Design review of the part built by this model. Coordinates are the model's own, in mm. A direction names the side the tool comes from. Coordinates: 2 decimals unless noted, no trailing zeros. Loops run counter-clockwise (first coordinate to the right, second up) from the corner with the lowest first, then second, coordinate; pieces in that order, holes last. Notation, with made-up numbers: (27.25, -2.5) -> (35.25, -2.5) arc R21 cw to (35.25, 4.5) -> close; hole circle Ø4 at (-2.5, 21.25). An arc over 180 degrees is marked (long way). Answer in a Markdown table with one row per item.
```python
from build123d import *

# Parameters (mm, degrees)
SKETCH1_R               = 63.5
BOSS_EXTRUDE1_DEPTH     = 25.4
SKETCH2_R               = 38.1
CUT_EXTRUDE1_DEPTH      = 12.7
BOSS_EXTRUDE2_DEPTH     = 50.8
SKETCH5_R               = 3.175
CUT_EXTRUDE2_DEPTH      = 1
CUT_EXTRUDE2_DEPTH_BACK = 77.2
SKETCH8_R               = 3.175
CUT_EXTRUDE3_DEPTH      = 15.24
SKETCH7_R               = 3.175
CUT_EXTRUDE5_DEPTH      = 15.24
SKETCH6_R               = 3.175
CUT_EXTRUDE6_DEPTH      = 15.24


with BuildPart() as part:
    # Sketch1 → Boss-Extrude1 (new body)
    with BuildSketch(Plane(origin=(0, 0, 0), x_dir=(1, 0, 0), z_dir=(0, 1, 0))):
        Circle(SKETCH1_R)
    extrude(amount=BOSS_EXTRUDE1_DEPTH)

    # Sketch2 → Cut-Extrude1 (cut)
    with BuildSketch(Plane(origin=(0, 25.4, 0), x_dir=(1, 0, 0), z_dir=(0, 1, 0))):
        Circle(SKETCH2_R)
    extrude(amount=-CUT_EXTRUDE1_DEPTH, mode=Mode.SUBTRACT)

    # Sketch4 → Boss-Extrude2 (add)
    with BuildSketch(Plane.XZ):
        Polygon((50.8, -29.329393675), (0, 58.65878735), (-50.8, -29.329393675), align=None)
    extrude(amount=BOSS_EXTRUDE2_DEPTH)

    # Sketch5 → Cut-Extrude2 (cut, two sides)
    with BuildSketch(Plane(origin=(0, 25.4, 0), x_dir=(1, 0, 0), z_dir=(0, 1, 0))) as cut_extrude2_sk:
        with Locations((0, 50.8)):
            Circle(SKETCH5_R)
        with Locations((43.994090512, -25.4)):
            Circle(SKETCH5_R)
        with Locations((-43.994090512, -25.4)):
            Circle(SKETCH5_R)
    extrude(amount=CUT_EXTRUDE2_DEPTH, mode=Mode.SUBTRACT)
    extrude(cut_extrude2_sk.sketch, amount=-CUT_EXTRUDE2_DEPTH_BACK, mode=Mode.SUBTRACT)

    # Sketch8 → Cut-Extrude3 (cut)
    with BuildSketch(Plane(origin=(-25.4, 0, 14.664696837), x_dir=(0.5, 0, 0.866025404), z_dir=(-0.866025404, 0, 0.5))):
        with Locations((0, -25.4)):
            Circle(SKETCH8_R)
    extrude(amount=-CUT_EXTRUDE3_DEPTH, mode=Mode.SUBTRACT)

    # Sketch7 → Cut-Extrude5 (cut)
    with BuildSketch(Plane(origin=(3.754579306, 0, -29.329393675), x_dir=(1, 0, 0), z_dir=(0, 0, 1))):
        with Locations((-3.754579306, -25.4)):
            Circle(SKETCH7_R)
    extrude(amount=CUT_EXTRUDE5_DEPTH, mode=Mode.SUBTRACT)

    # Sketch6 → Cut-Extrude6 (cut)
    with BuildSketch(Plane(origin=(25.4, 0, 14.664696837), x_dir=(0.5, 0, -0.866025404), z_dir=(0.866025404, 0, 0.5))):
        with Locations((0, -25.4)):
            Circle(SKETCH6_R)
    extrude(amount=-CUT_EXTRUDE6_DEPTH, mode=Mode.SUBTRACT)


solid = part.part
```
(1) Draft analysis for pull direction Z (two halves, no side actions). For faces 1 (the flat face through (27.3, 25.4, 27.3)), 2 (the flat face through (-12.22, -25.36, 7.01)), 3 (the cylindrical face through (-13.77, 12.52, 61.99)), 4 (the flat face through (-1, -31, -29.329)), state which applies: pulls with the +Z half, pulls with the -Z half, needs draft (parallel to the pull), parting line crosses it, or undercut.
Evaluation:
| item | result |
|---|---|
| face 1 | needs draft |
| face 2 | undercut |
| face 3 | parting line crosses it |
| face 4 | pulls with the -Z half |
(2) Take a section at C-C on y = -45.5. Give the boundary of the cut face in (x, z), and give its area (3 significant figures).
Evaluation:
| item | result |
|---|---|
| outline | (-50.8, -29.33) -> (50.8, -29.33) -> (0, 58.66) -> close |
| area | 4,470 mm² |
(3) For pin 1 (10 mm diameter, centred on x = 0, z = -50.8, fed in from -Y); pin 2 (8 mm diameter, centred on y = 6.5, z = 15.5, fed in from -X); pin 3 (12 mm diameter, centred on x = 30, y = 12.5, fed in from -Z); pin 4 (10 mm diameter, centred on x = -43.99, z = 25.4, fed in from +Y), all flat-tipped, find the tip position at first contact; note any pin that passes through.
Evaluation:
| item | result |
|---|---|
| pin 1 | stops at y = 0 |
| pin 2 | stops at x = -62.45 |
| pin 3 | stops at z = -58.79 |
| pin 4 | stops at y = 25.4 |
(4) Take a section at D-D on z = 0. Give the boundary of the cut face in (x, y), and give its area (3 significant figures).
Evaluation:
| item | result |
|---|---|
| outline | (-63.5, 0) -> (-33.87, 0) -> (-33.87, -50.8) -> (33.87, -50.8) -> (33.87, 0) -> (63.5, 0) -> (63.5, 25.4) -> (38.1, 25.4) -> (38.1, 12.7) -> (-38.1, 12.7) -> (-38.1, 25.4) -> (-63.5, 25.4) -> close |
| area | 5,700 mm² |
(5) Take a section at B-B on z = 25.4. Give the boundary of the cut face in (x, y).
Evaluation:
| item | result |
|---|---|
| outline | (-58.2, 0) -> (-47.17, 0) -> (-47.17, 25.4) -> (-58.2, 25.4) -> close; (-40.82, 0) -> (-19.2, 0) -> (-19.2, -50.8) -> (19.2, -50.8) -> (19.2, 0) -> (40.82, 0) -> (40.82, 25.4) -> (28.4, 25.4) -> (28.4, 12.7) -> (-28.4, 12.7) -> (-28.4, 25.4) -> (-40.82, 25.4) -> close; (47.17, 0) -> (58.2, 0) -> (58.2, 25.4) -> (47.17, 25.4) -> close |
(6) To check wall thickness, follow probe 1 along Z at (x, y) = (0, 19.5) (3 decimals); probe 2 along X at (y, z) = (9.25, 25.4); probe 3 along Y at (x, z) = (0, -26) (3 decimals). State the ranges of each line that lie inside material, in increasing order.
Evaluation:
| item | result |
|---|---|
| probe 1 | z = -63.5 to -53.975, -47.625 to -38.1, 38.1 to 63.5 |
| probe 2 | x = -58.2 to -47.17, -40.82 to 40.82, 47.17 to 58.2 |
| probe 3 | y = -50.8 to -28.575, -22.225 to 12.7 |
(7) Tool access review of faces 5 (the cylindrical face through (-0.41, -22.25, -21.82)), 6 (the flat face through (-1, 12.7, -1)), 7 (the flat face through (-25.044, -30.689, 15.281)): name each direction out of +Z, -Z, +X, -X, +Y, -Y from which nothing blocks a thin tool from reaching the whole face with its end or side.
Evaluation:
| item | result |
|---|---|
| face 5 | -Z |
| face 6 | +Y |
| face 7 | +Z, -X, -Y |
(8) Take a section at A-A on z = -50.8. Give the boundary of the cut face in (x, y) (3 decimals).
Evaluation:
| item | result |
|---|---|
| outline | (-38.1, 0) -> (-3.175, 0) -> (-3.175, 25.4) -> (-38.1, 25.4) -> close; (3.175, 0) -> (38.1, 0) -> (38.1, 25.4) -> (3.175, 25.4) -> close |
